from build123d import *

# Parameters (mm, degrees)
SKETCH_1_W          = 27.399999997
SKETCH_1_H          = 4
EXTRUDE_1_DEPTH     = 3
SKETCH_1_3_W        = 27.399999997
SKETCH_1_3_H        = 4
EXTRUDE_2_DEPTH     = 11
SKETCH_1_4_W        = 27.399999997
SKETCH_1_4_H        = 4
EXTRUDE_3_DEPTH     = 8
SKETCH_2_R          = 1.5
CUT_EXTRUDE_1_DEPTH = 6.5
FILLET_1_R          = 4
EXTRUDE_4_DEPTH     = 19
SKETCH_6_W          = 32.257266432
SKETCH_6_H          = 23.708854684
CUT_EXTRUDE_2_DEPTH = 21
SKETCH_7_W          = 8
SKETCH_7_H          = 4
EXTRUDE_5_DEPTH     = 5
SKETCH_8_W          = 8
SKETCH_8_H          = 4
EXTRUDE_6_DEPTH     = 5
FILLET_2_R          = 5


with BuildPart() as part:
    # 草图1 → 凸台-拉伸1 (new body)
    with BuildSketch(Plane.XY):
        with BuildLine():
            ThreePointArc((-0.337371922, -1.853501365), (-0.488220409, -1.87454383), (-0.640366957, -1.881577989))
            Line((-0.640366957, -1.881577989), (-1.640366957, -1.881577989))
            Line((-1.640366957, -1.881577989), (-1.640366957, -2.881577989))
            Line((-1.640366957, -2.881577989), (25.75963304, -2.881577989))
            Line((25.75963304, -2.881577989), (25.75963304, -1.88157799))
            Line((25.75963304, -1.88157799), (24.75963304, -1.88157799))
            ThreePointArc((24.75963304, -1.88157799), (24.607486492, -1.87454383), (24.456638005, -1.853501365))
            ThreePointArc((24.456638005, -1.853501365), (23.608703525, -1.413476758), (23.147062635, -0.577114262))
            ThreePointArc((23.147062635, -0.577114262), (22.880535784, 0.365382964), (22.493851477, 1.265278974))
            ThreePointArc((22.493851477, 1.265278974), (21.584633042, 1.287629087), (20.675414607, 1.265278974))
            ThreePointArc((20.675414607, 1.265278974), (20.288730299, 0.365382964), (20.022203448, -0.577114261))
            ThreePointArc((20.022203448, -0.577114261), (19.560562558, -1.413476758), (18.712628078, -1.853501365))
            ThreePointArc((18.712628078, -1.853501365), (18.409633042, -1.88157799), (18.106638005, -1.853501365))
            ThreePointArc((18.106638005, -1.853501365), (17.258703525, -1.413476758), (16.797062635, -0.577114262))
            ThreePointArc((16.797062635, -0.577114262), (16.530535784, 0.365382964), (16.143851477, 1.265278974))
            ThreePointArc((16.143851477, 1.265278974), (15.234633042, 1.287629087), (14.325414607, 1.265278974))
            ThreePointArc((14.325414607, 1.265278974), (13.938730299, 0.365382964), (13.672203448, -0.577114261))
            ThreePointArc((13.672203448, -0.577114261), (13.210562558, -1.413476758), (12.362628078, -1.853501365))
            ThreePointArc((12.362628078, -1.853501365), (12.059633042, -1.88157799), (11.756638005, -1.853501365))
            ThreePointArc((11.756638005, -1.853501365), (10.908703525, -1.413476758), (10.447062635, -0.577114262))
            ThreePointArc((10.447062635, -0.577114262), (10.180535784, 0.365382964), (9.793851477, 1.265278974))
            ThreePointArc((9.793851477, 1.265278974), (8.884633042, 1.287629087), (7.975414607, 1.265278974))
            ThreePointArc((7.975414607, 1.265278974), (7.588730299, 0.365382964), (7.322203448, -0.577114261))
            ThreePointArc((7.322203448, -0.577114261), (6.860562558, -1.413476758), (6.012628078, -1.853501365))
            ThreePointArc((6.012628078, -1.853501365), (5.709633042, -1.88157799), (5.406638005, -1.853501365))
            ThreePointArc((5.406638005, -1.853501365), (4.558703525, -1.413476758), (4.097062635, -0.577114262))
            ThreePointArc((4.097062635, -0.577114262), (3.830535784, 0.365382964), (3.443851477, 1.265278974))
            ThreePointArc((3.443851477, 1.265278974), (2.534633042, 1.287629087), (1.625414607, 1.265278974))
            ThreePointArc((1.625414607, 1.265278974), (1.238730299, 0.365382964), (0.972203448, -0.577114261))
            ThreePointArc((0.972203448, -0.577114261), (0.510562558, -1.413476758), (-0.337371922, -1.853501365))
        make_face()
        with Locations((12.059633041, -4.881577989)):
            Rectangle(SKETCH_1_W, SKETCH_1_H)
    extrude(amount=EXTRUDE_1_DEPTH)

    # 草图1<3> → 凸台-拉伸2 (add)
    with BuildSketch(Plane.XY):
        with Locations((12.059633041, -4.881577989)):
            Rectangle(SKETCH_1_3_W, SKETCH_1_3_H)
    extrude(amount=EXTRUDE_2_DEPTH)

    # 草图1<4> → 凸台-拉伸3 (add)
    with BuildSketch(Plane.XY):
        with Locations((12.059633041, -4.881577989)):
            Rectangle(SKETCH_1_4_W, SKETCH_1_4_H)
    extrude(amount=-EXTRUDE_3_DEPTH)

    # 草图2 → 切除-拉伸1 (cut)
    with BuildSketch(Plane(origin=(0, -2.881577989, 0), x_dir=(1, 0, 0), z_dir=(0, 1, 0))):
        with Locations(Location((2.059633042, 4.5, 0), (0, 0, 270))):
            Circle(SKETCH_2_R)
        with Locations(Location((22.059633042, 4.5, 0), (0, 0, 270))):
            Circle(SKETCH_2_R)
        with Locations(Location((22.059633042, -7.5, 0), (0, 0, 270))):
            Circle(SKETCH_2_R)
        with Locations(Location((2.059633042, -7.5, 0), (0, 0, 270))):
            Circle(SKETCH_2_R)
    extrude(amount=-CUT_EXTRUDE_1_DEPTH, mode=Mode.SUBTRACT)

    # 圆角1
    fillet_1_edges = [part.edges().sort_by_distance(p)[0] for p in [
        (25.75963304, -4.881577989, 11),
        (25.75963304, -4.881577989, -8),
    ]]
    fillet(fillet_1_edges, radius=FILLET_1_R)

    # 草图4 → 凸台-拉伸4 (add)
    with BuildSketch(Plane(origin=(0, 0, -8), x_dir=(-1, 0, 0), z_dir=(0, 0, -1))):
        with BuildLine():
            Line((-7.559633042, -6.881577989), (-12.559633042, -6.881577989))
            Line((-12.559633042, -6.881577989), (-12.559633042, -12.881577989))
            ThreePointArc((-12.559633042, -12.881577989), (-9.530706272, -19.615542978), (-2.482680937, -21.816910897))
            Line((-2.482680937, -21.816910897), (-2.482680937, -19.612245623))
            ThreePointArc((-2.482680937, -19.612245623), (-6.148073578, -17.096946581), (-7.559633042, -12.881577989))
            Line((-7.559633042, -12.881577989), (-7.559633042, -6.881577989))
        make_face()
    extrude(amount=-EXTRUDE_4_DEPTH)

    # 草图6 → 切除-拉伸2 (cut)
    with BuildSketch(Plane.XZ.offset(6.881577989)):
        with Locations((13.405653676, 0.508195322)):
            Rectangle(SKETCH_6_W, SKETCH_6_H)
    extrude(amount=CUT_EXTRUDE_2_DEPTH, mode=Mode.SUBTRACT)

    # 草图7 → 凸台-拉伸5 (add)
    with BuildSketch(Plane.XY.offset(11)):
        with Locations((2.359633043, -4.881577989)):
            Rectangle(SKETCH_7_W, SKETCH_7_H)
    extrude(amount=EXTRUDE_5_DEPTH)

    # 草图8 → 凸台-拉伸6 (add)
    with BuildSketch(Plane(origin=(0, 0, -8), x_dir=(-1, 0, 0), z_dir=(0, 0, -1))):
        with Locations((-2.359633043, -4.881577989)):
            Rectangle(SKETCH_8_W, SKETCH_8_H)
    extrude(amount=EXTRUDE_6_DEPTH)

    # 圆角2
    fillet_2_edges = [part.edges().sort_by_distance(p)[0] for p in [
        (6.359633043, -4.881577989, 11),
        (6.359633043, -4.881577989, -8),
    ]]
    fillet(fillet_2_edges, radius=FILLET_2_R - 0.0001)  # a hair under: the kernel refuses the full size


solid = part.part
Here's how the part is built. I have some questions about the finished solid (model axes, mm). A direction names the side the tool comes from. Give positions to 0.01 mm unless a question says otherwise; leave off trailing zeros. Order: outer loops, then holes, each group sorted by start corner. A loop starts at its lowest first (then second) coordinate and runs counter-clockwise, first axis right, second up. Notation, with made-up numbers: (70, 26.5) -> (125, 26.5) arc R23 cw to (125, 65.5) -> close; hole circle Ø7 at (50.25, 21). An arc over 180 degrees is marked (long way). One line per item, written item: value. Start each with the question number.
1. Imagine slicing it at B-B, the plane z = 1.75. List the corners of the cut face in (x, y) for me (1 decimal).
2. Imagine slicing it at D-D, the plane y = -6. Count the separate pieces of the cut face and the enclosed holes in it, plus the area to 3 significant figures.
3. For faces 1 (the face through (13.943, 0.378, 1.479)), 2 (the face through (9, -2.882, -5)), 3 (the face through (25.76, -5, 2)), which set-ups out of +Z, -Z, +X, -X, +Y, -Y let a thin tool reach every point of the face, with its end or its side?
4. I need wall thicknesses on probe 1 along Z at (x, y) = (3.25, -3); probe 2 along Z at (x, y) = (3, 1.25); probe 3 along Y at (x, z) = (3, 13.25). Which ranges of each line are inside material? Lowest first, please. Write a range as from..to.
5. Imagine slicing it at A-A, the plane y = 0.25. List the corners of the cut face in (x, z) for me, plus the area to 3 significant figures.
6. Will these pins go through, and if not, where does the flat tip stop? pin 1 Ø3.5 at (x, y) = (13.5, -1.5) entering from -Z; pin 2 Ø1.3 at (x, y) = (6, -1.5) entering from +Z; pin 3 Ø0.5 at (x, z) = (-1, 1) entering from +Y; pin 4 Ø1.8 at (x, z) = (22.06, 7.5) entering from -Y.
7. Imagine slicing it at C-C, the plane z = 7.5. List the corners of the cut face in (x, y) for me, plus the area to 3 significant figures.
8. We'd pull the mould along Z, two halves only. Please class faces 4 (the face through (16, -5, -8)), 5 (the face through (11.9, -2.2, 3)), 6 (the face through (25, -1.882, 1)), 7 (the face through (0.595, -4.854, -4.825)): released by +Z, released by -Z, zero draft, split by the parting line, or undercut.
Values follow:
1. outline: (-1.6, -6.9) -> (25.8, -6.9) -> (25.8, -1.9) -> (24.8, -1.9) arc R1.6 cw to (23.1, -0.6) arc R7.5 ccw to (22.5, 1.3) arc R18.5 ccw to (20.7, 1.3) arc R7.5 ccw to (20, -0.6) arc R1.6 cw to (16.8, -0.6) arc R7.5 ccw to (16.1, 1.3) arc R18.5 ccw to (14.3, 1.3) arc R7.5 ccw to (13.7, -0.6) arc R1.6 cw to (10.4, -0.6) arc R7.5 ccw to (9.8, 1.3) arc R18.5 ccw to (8, 1.3) arc R7.5 ccw to (7.3, -0.6) arc R1.6 cw to (4.1, -0.6) arc R7.5 ccw to (3.4, 1.3) arc R18.5 ccw to (1.6, 1.3) arc R7.5 ccw to (1, -0.6) arc R1.6 cw to (-0.6, -1.9) -> (-1.6, -1.9) -> close
2. separate pieces: 1
2. enclosed holes: 4
2. area: 576 mm2
3. face 1: +Z, -Z, +Y
3. face 2: -Z, +X, -X, +Y
3. face 3: +Z, -Z, +X, +Y, -Y
4. probe 1: z = -13..-5.41, -3.59..6.59, 8.41..16
4. probe 2: z = 0..3
4. probe 3: y = -6.88..-2.88
5. outline: (1.2, 0) -> (3.87, 0) -> (3.87, 3) -> (1.2, 3) -> close; (7.55, 0) -> (10.22, 0) -> (10.22, 3) -> (7.55, 3) -> close; (13.9, 0) -> (16.57, 0) -> (16.57, 3) -> (13.9, 3) -> close; (20.25, 0) -> (22.92, 0) -> (22.92, 3) -> (20.25, 3) -> close
5. area: 32.1 mm2
6. pin 1: stops at z = -8
6. pin 2: stops at z = 3
6. pin 3: stops at y = -1.88
6. pin 4: passes through
7. outline: (-1.64, -6.88) -> (0.56, -6.88) -> (0.56, -2.88) -> (-1.64, -2.88) -> close; (3.56, -6.88) -> (20.56, -6.88) -> (20.56, -2.88) -> (3.56, -2.88) -> close; (23.56, -6.88) -> (25.73, -6.88) -> (25.73, -2.88) -> (23.56, -2.88) -> close
7. area: 85.5 mm2
8. face 4: released by -Z
8. face 5: released by +Z
8. face 6: zero draft
8. face 7: undercut
